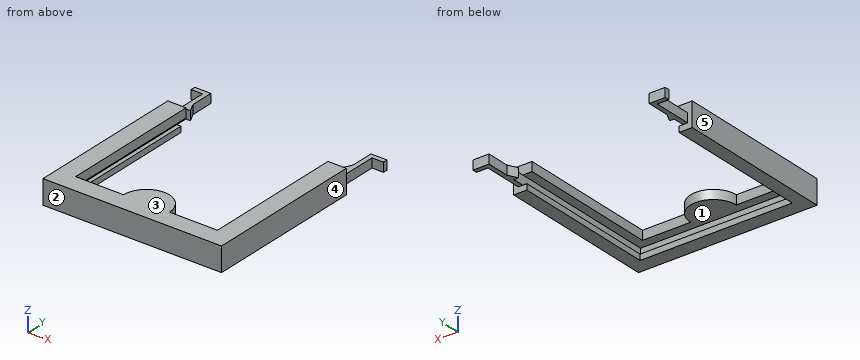
from build123d import *

# Parameters (mm, degrees)
BOSS_EXTRU_1_DEPTH = 6.5
BOSS_EXTRU_2_DEPTH = 2.5
ESQUISSE3_W        = 2
ESQUISSE3_H        = 4
BOSS_EXTRU_3_DEPTH = 9
BOSS_EXTRU_4_START = -4
BOSS_EXTRU_4_DEPTH = 4
BOSS_EXTRU_5_DEPTH = 4
ESQUISSE6_W        = 2
ESQUISSE6_H        = 4
BOSS_EXTRU_6_DEPTH = 10
ESQUISSE7_W        = 4
ESQUISSE7_H        = 2
BOSS_EXTRU_7_DEPTH = 5
ESQUISSE8_W        = 4
ESQUISSE8_H        = 2
BOSS_EXTRU_8_DEPTH = 5
BOSS_EXTRU_9_START = -4
BOSS_EXTRU_9_DEPTH = 4


with BuildPart() as part:
    # Esquisse1 → Boss.-Extru.1 (new body)
    with BuildSketch(Plane.XY):
        Polygon((-74, 4), (-74, 70), (-78, 70), (-78, 0), (0, 0), (0, 70), (-4, 70), (-4, 4), align=None)
    extrude(amount=BOSS_EXTRU_1_DEPTH)

    # Esquisse2 → Boss.-Extru.2 (add)
    with BuildSketch(Plane(origin=(0, 0, 0), x_dir=(-1, 0, 0), z_dir=(0, 0, -1))):
        Polygon((0, 70), (5.75, 70), (5.75, 6.5), (72.25, 6.5), (72.25, 70), (78, 70), (78, 0), (0, 0), align=None)
    extrude(amount=-BOSS_EXTRU_2_DEPTH)

    # Esquisse3 → Boss.-Extru.3 (add)
    with BuildSketch(Plane(origin=(0, 70, 0), x_dir=(1, 0, 0), z_dir=(0, 1, 0))):
        with Locations((-75, -4.5)):
            Rectangle(ESQUISSE3_W, ESQUISSE3_H)
        with Locations((-3, -4.5)):
            Rectangle(ESQUISSE3_W, ESQUISSE3_H)
    extrude(amount=BOSS_EXTRU_3_DEPTH)

    # Esquisse4 → Boss.-Extru.4 (add)
    with BuildSketch(Plane.XY.offset(6.5).offset(BOSS_EXTRU_4_START)):
        Polygon((-4, 79), (-6, 75), (-4, 75), align=None)
        Polygon((-74, 79), (-72, 75), (-74, 75), align=None)
    extrude(amount=BOSS_EXTRU_4_DEPTH)

    # Esquisse5 → Boss.-Extru.5 (add)
    with BuildSketch(Plane.XY.offset(6.5)):
        Polygon((0, 70), (0, 0), (-78, 0), (-78, 70), (-70, 70), (-70, 8), (-8, 8), (-8, 70), align=None)
    extrude(amount=BOSS_EXTRU_5_DEPTH)

    # Esquisse6 → Boss.-Extru.6 (add)
    with BuildSketch(Plane(origin=(0, 79, 0), x_dir=(1, 0, 0), z_dir=(0, 1, 0))):
        with Locations((-3, -4.5)):
            Rectangle(ESQUISSE6_W, ESQUISSE6_H)
        with Locations((-75, -4.5)):
            Rectangle(ESQUISSE6_W, ESQUISSE6_H)
    extrude(amount=BOSS_EXTRU_6_DEPTH)

    # Esquisse7 → Boss.-Extru.7 (add)
    with BuildSketch(Plane(origin=(-2, 0, 0), x_dir=(0, 0, -1), z_dir=(1, 0, 0))):
        with Locations((-4.5, 88)):
            Rectangle(ESQUISSE7_W, ESQUISSE7_H)
    extrude(amount=BOSS_EXTRU_7_DEPTH)

    # Esquisse8 → Boss.-Extru.8 (add)
    with BuildSketch(Plane.ZY.offset(76)):
        with Locations((4.5, 88)):
            Rectangle(ESQUISSE8_W, ESQUISSE8_H)
    extrude(amount=BOSS_EXTRU_8_DEPTH)

    # Esquisse9 → Boss.-Extru.9 (add)
    with BuildSketch(Plane.XY.offset(10.5).offset(BOSS_EXTRU_9_START)):
        with BuildLine():
            Line((-49, 8), (-29, 8))
            ThreePointArc((-29, 8), (-39, 18), (-49, 8))
        make_face()
    extrude(amount=BOSS_EXTRU_9_DEPTH)


solid = part.part
Can you work these out from the model? Positions are in its coordinate system, mm. Face numbers are marked on the shaded views. A direction names the side the tool comes from. Give positions to 0.01 mm unless a question says otherwise; leave off trailing zeros. Write each loop counter-clockwise with the first axis right and the second up, starting at its lowest first coordinate (ties: lowest second). Pieces come first, ordered by that corner, then holes. Notation, with made-up numbers: (-11, 76.25) -> (11, 76.25) arc R19 cw to (11, 98.25) -> close; hole circle Ø5 at (21, -33.5). An arc over 180 degrees is marked (long way). Answer as a JSON object with one key per item and string values. Group by question number.
Item 1: I'm going to push flat-ended pins straight in: P1, Ø0.8, axis at y = 51, z = 1, coming from the -X side; P2, Ø1.2, axis at x = -59, z = 9, coming from the +Y side; P3, Ø4.5, axis at y = 83.5, z = 5, coming from the -X side. Where does each tip first touch, or does it pass through?
Item 2: Suppose I cut it at B-B (x = -39). Please give me the cut outline in (y, z).
Item 3: For the marked faces 4 and 5, which set-ups out of +Z, -Z, +X, -X, +Y, -Y let a thin tool reach every point of the face, with its end or its side?
Item 4: We'd pull the mould along Z, two halves only. Please class the marked faces 1, 2 and 3: +Z half, -Z half, draft (parallel to the pull), parting line (faces both ways), or undercut.
Item 5: Please list where these lines run through material, in increasing order: line 1 (X direction, y = 29, z = 6.25); line 2 (X direction, y = 43, z = 7.75); line 3 (Y direction, x = -58, z = 9). Write a range as [from, to].
Item 6: Suppose I cut it at D-D (x = -22). Please give me the cut outline in (y, z), plus the area to 4 significant figures.
Item 7: Suppose I cut it at A-A (y = 65). Please give me the cut outline in (x, z), plus the area to 3 significant figures.
Item 8: Suppose I cut it at C-C (z = 4.75). Please give me the cut outline in (x, y).
Findings:
{
 "1": {"P1": "stops at x = -78", "P2": "stops at y = 8", "P3": "stops at x = -76"},
 "2": {"outline": "(0, 0) -> (6.5, 0) -> (6.5, 2.5) -> (4, 2.5) -> (4, 6.5) -> (18, 6.5) -> (18, 10.5) -> (0, 10.5) -> close"},
 "3": {"face 4": "+Z, -Z, +X, -Y", "face 5": "+Z, -Z, -X, -Y"},
 "4": {"face 1": "undercut", "face 2": "draft", "face 3": "+Z half"},
 "5": {"line 1": "x = [-78, -74], [-4, 0]", "line 2": "x = [-78, -70], [-8, 0]", "line 3": "y = [0, 8]"},
 "6": {"outline": "(0, 0) -> (6.5, 0) -> (6.5, 2.5) -> (4, 2.5) -> (4, 6.5) -> (8, 6.5) -> (8, 10.5) -> (0, 10.5) -> close", "area": "64.25 mm²"},
 "7": {"outline": "(-78, 0) -> (-72.25, 0) -> (-72.25, 2.5) -> (-74, 2.5) -> (-74, 6.5) -> (-70, 6.5) -> (-70, 10.5) -> (-78, 10.5) -> close; (-8, 6.5) -> (-4, 6.5) -> (-4, 2.5) -> (-5.75, 2.5) -> (-5.75, 0) -> (0, 0) -> (0, 10.5) -> (-8, 10.5) -> close", "area": "125 mm²"},
 "8": {"outline": "(-81, 87) -> (-76, 87) -> (-76, 70) -> (-78, 70) -> (-78, 0) -> (0, 0) -> (0, 70) -> (-2, 70) -> (-2, 87) -> (3, 87) -> (3, 89) -> (-4, 89) -> (-4, 79) -> (-6, 75) -> (-4, 75) -> (-4, 4) -> (-74, 4) -> (-74, 75) -> (-72, 75) -> (-74, 79) -> (-74, 89) -> (-81, 89) -> close"}
}
